from build123d import *

# Parameters (mm, degrees)
FRAME_EXTERIOR_MASTER_OUTLINE_R = 19.685
FRAME_EXTERIOR_MASTER_DEPTH     = 6.35
CUT_EXTRUDE1_DEPTH              = 611.690430988


# Read off the part's stored shape, not the designer's step: Frame Exterior Master
with BuildPart() as part:
    # Frame Exterior Master outline → Frame Exterior Master (new body)
    with BuildSketch(Plane.XY):
        Polygon((431.8, 12.7), (431.8, 431.8), (215.9, 431.8), (0, 304.8), (0, 12.7), (127, 12.7), (127, 50.8), (254, 50.8), (254, 12.7), align=None)
        with Locations((98.15, 150.3)):
            Circle(FRAME_EXTERIOR_MASTER_OUTLINE_R, mode=Mode.SUBTRACT)
        with Locations((333.65, 150.3)):
            Circle(FRAME_EXTERIOR_MASTER_OUTLINE_R, mode=Mode.SUBTRACT)
    extrude(amount=FRAME_EXTERIOR_MASTER_DEPTH)

    # Sketch1 → Cut-Extrude1 (cut, through all)
    with BuildSketch(Plane.XY.offset(6.35)):
        Polygon((127, 298.45), (127, 57.15), (254, 57.15), (254, 171.45), (355.6, 171.45), (355.6, 298.45), align=None)
    extrude(amount=-CUT_EXTRUDE1_DEPTH, mode=Mode.SUBTRACT)


solid = part.part
Build history of the part. All positions in model axes, mm. Round coordinates to 2 decimals unless told otherwise and drop trailing zeros. Loops run counter-clockwise (first coordinate to the right, second up) from the corner with the lowest first, then second, coordinate; pieces in that order, holes last. Notation, with made-up numbers: (74.5, -31.5) -> (100.5, -31.5) arc R23 cw to (100.5, 0.5) -> close; hole circle Ø6 at (-12, 17). An arc over 180 degrees is marked (long way). Use CSV: the item, a comma, the result in double quotes. Start each with the question number.
Q1. Saw through at A-A on x = 333.65. Give the cut face in (y, z) (3 decimals), and give its area (3 significant figures).
Q2. Drill centre lines: L1, parallel to Y at x = 332, z = 6; L2, parallel to Y at x = 333.65, z = 1.75 (3 decimals); L3, parallel to Y at x = 244, z = 4.5. Where is each one in solid material? Low to high.
Q3. Flat gauge pins, fed straight in: pin 1 Ø2 at (y, z) = (321.5, 3) entering from -X; pin 2 Ø23.5 at (x, y) = (333.65, 150.3) entering from +Z. Where does each tip first touch, or does it go through?
Q4. Mould opens along X. For faces 1 (the face through (261, 132, 0)), 2 (the face through (109.46, 369.19, 3.13)), 3 (the face through (331.087, 169.817, 3.131)) say: +X half, -X half, draft (parallel to the pull), parting line (faces both ways), or undercut.
Q5. Saw through at B-B on y = 288.5. Give the cut face in (x, z).
Q6. Saw through at D-D on z = 1. Give the cut face in (x, y) (3 decimals).
Q7. Saw through at C-C on x = 243. Give the cut face in (y, z), and give its area (3 significant figures).
Solutions:
1,outline,"(12.7, 0) -> (130.615, 0) -> (130.615, 6.35) -> (12.7, 6.35) -> close; (169.985, 0) -> (171.45, 0) -> (171.45, 6.35) -> (169.985, 6.35) -> close; (298.45, 0) -> (431.8, 0) -> (431.8, 6.35) -> (298.45, 6.35) -> close"
1,area,"1,600 mm^2"
2,L1,"y = 12.7 to 130.68, 169.92 to 171.45, 298.45 to 431.8"
2,L2,"y = 12.7 to 130.615, 169.985 to 171.45, 298.45 to 431.8"
2,L3,"y = 50.8 to 57.15, 298.45 to 431.8"
3,pin 1,"stops at x = 26.69"
3,pin 2,"passes through"
4,face 1,"draft"
4,face 2,"-X half"
4,face 3,"undercut"
5,outline,"(0, 0) -> (127, 0) -> (127, 6.35) -> (0, 6.35) -> close; (355.6, 0) -> (431.8, 0) -> (431.8, 6.35) -> (355.6, 6.35) -> close"
6,outline,"(0, 12.7) -> (127, 12.7) -> (127, 50.8) -> (254, 50.8) -> (254, 12.7) -> (431.8, 12.7) -> (431.8, 431.8) -> (215.9, 431.8) -> (0, 304.8) -> close; hole circle Ø39.37 at (98.15, 150.3); hole (127, 57.15) -> (254, 57.15) -> (254, 171.45) -> (355.6, 171.45) -> (355.6, 298.45) -> (127, 298.45) -> close; hole circle Ø39.37 at (333.65, 150.3)"
7,outline,"(50.8, 0) -> (57.15, 0) -> (57.15, 6.35) -> (50.8, 6.35) -> close; (298.45, 0) -> (431.8, 0) -> (431.8, 6.35) -> (298.45, 6.35) -> close"
7,area,"887 mm^2"
